Verification items for the finished model (mm, model axes). Face numbers are marked on the shaded views. A direction names the side the tool comes from. Round coordinates to 2 decimals unless told otherwise and drop trailing zeros. Loops run counter-clockwise (first coordinate to the right, second up) from the corner with the lowest first, then second, coordinate; pieces in that order, holes last. Notation, with made-up numbers: M -34.75,-4 L -15.75,-4 A25 cw -15.75,12 Z; hole C 34,-1.75 d11. An arc over 180 degrees is marked long. One line per item, written item: value.
from build123d import *

# Parameters (mm, degrees)
SKIZZE1_W                       = 60
SKIZZE1_H                       = 70
GRUNDK_RPER_DEPTH               = 20
FASE1_SIZE                      = 2
WANDUNG1_T                      = 3
SKIZZE2_R                       = 4.5
DURCHBRUCH_SERVO_DEPTH          = 100.13122616
SKIZZE4_W                       = 22
SKIZZE4_H                       = 42
SERVOFREISCHNITT_DEPTH          = 2
SKIZZE3_R                       = 2.1
FLANSCHAUFSATZ_DEPTH            = 6.5
SKIZZE6_R                       = 17.125
BOHRUNGSCHNECKE_DEPTH           = 6.5
SCHNITT_LINEAR_AUSTRAGEN2_REACH = 101.131
SKIZZE7_R                       = 2
SKIZZE8_R                       = 3.6
SCHNITT_LINEAR_AUSTRAGEN3_DEPTH = 2
FASE2_SIZE                      = 1
FASE3_SIZE                      = 0.5


with BuildPart() as part:
    # Skizze1 → Grundkörper (new body)
    with BuildSketch(Plane.XY):
        with Locations((30, 35)):
            Rectangle(SKIZZE1_W, SKIZZE1_H)
    extrude(amount=GRUNDK_RPER_DEPTH)

    # Fase1
    fase1_edges = [part.edges().sort_by_distance(p)[0] for p in [
        (0, 70, 10),
        (60, 70, 10),
        (60, 0, 10),
        (0, 0, 10),
    ]]
    chamfer(fase1_edges, length=FASE1_SIZE)

    # Wandung1
    wandung1_openings = [part.faces().sort_by_distance(p)[0] for p in [
        (30, 35, 0),
    ]]
    offset(amount=WANDUNG1_T, openings=wandung1_openings, kind=Kind.INTERSECTION)

    # Skizze2 → Durchbruch Servo (cut, through all)
    with BuildSketch(Plane.XY.offset(23)):
        with Locations((30, 24)):
            Circle(SKIZZE2_R)
    extrude(amount=-DURCHBRUCH_SERVO_DEPTH, mode=Mode.SUBTRACT)

    # Skizze4 → ServoFreischnitt (cut)
    with BuildSketch(Plane(origin=(0, 0, 20), x_dir=(-1, 0, 0), z_dir=(0, 0, -1))):
        with Locations((-30, 35)):
            Rectangle(SKIZZE4_W, SKIZZE4_H)
    extrude(amount=-SERVOFREISCHNITT_DEPTH, mode=Mode.SUBTRACT)

    # Skizze3 → FlanschAufsatz (add)
    with BuildSketch(Plane.XY.offset(23)):
        with BuildLine():
            Line((5, 31), (18.11121742, 38.820824834))
            ThreePointArc((18.11121742, 38.820824834), (30, 43), (41.88878258, 38.820824834))
            Line((41.88878258, 38.820824834), (55, 31))
            ThreePointArc((55, 31), (62, 24), (55, 17))
            Line((55, 17), (41.88878258, 9.179175166))
            ThreePointArc((41.88878258, 9.179175166), (30, 5), (18.11121742, 9.179175166))
            Line((18.11121742, 9.179175166), (5, 17))
            ThreePointArc((5, 17), (-2, 24), (5, 31))
        make_face()
        with Locations(Location((5, 24, 0), (0, 0, 180))):
            Circle(SKIZZE3_R, mode=Mode.SUBTRACT)
        with Locations(Location((55, 24, 0), (0, 0, 180))):
            Circle(SKIZZE3_R, mode=Mode.SUBTRACT)
    extrude(amount=FLANSCHAUFSATZ_DEPTH)

    # Skizze6 → BohrungSchnecke (cut)
    with BuildSketch(Plane.XY.offset(29.5)):
        with Locations((30, 24)):
            Circle(SKIZZE6_R)
    extrude(amount=-BOHRUNGSCHNECKE_DEPTH, mode=Mode.SUBTRACT)

    # Skizze7 → Schnitt-Linear austragen2 (cut, up to next)
    with BuildSketch(Plane.XY.offset(23), mode=Mode.PRIVATE) as schnitt_linear_austragen2_sk1:
        with Locations((8, 62)):
            Circle(SKIZZE7_R)
    schnitt_linear_austragen2_tool1 = extrude(schnitt_linear_austragen2_sk1.sketch, amount=-SCHNITT_LINEAR_AUSTRAGEN2_REACH, mode=Mode.PRIVATE) & part.part
    # Skizze7 → Schnitt-Linear austragen2 (cut, up to next)
    with BuildSketch(Plane.XY.offset(23), mode=Mode.PRIVATE) as schnitt_linear_austragen2_sk2:
        with Locations(Location((52, 62, 0), (0, 0, 180))):
            Circle(SKIZZE7_R)
    schnitt_linear_austragen2_tool2 = extrude(schnitt_linear_austragen2_sk2.sketch, amount=-SCHNITT_LINEAR_AUSTRAGEN2_REACH, mode=Mode.PRIVATE) & part.part
    # Skizze7 → Schnitt-Linear austragen2 (cut, up to next)
    with BuildSketch(Plane.XY.offset(23), mode=Mode.PRIVATE) as schnitt_linear_austragen2_sk3:
        with Locations((52, 8)):
            Circle(SKIZZE7_R)
    schnitt_linear_austragen2_tool3 = extrude(schnitt_linear_austragen2_sk3.sketch, amount=-SCHNITT_LINEAR_AUSTRAGEN2_REACH, mode=Mode.PRIVATE) & part.part
    # Skizze7 → Schnitt-Linear austragen2 (cut, up to next)
    with BuildSketch(Plane.XY.offset(23), mode=Mode.PRIVATE) as schnitt_linear_austragen2_sk4:
        with Locations(Location((8, 8, 0), (0, 0, 180))):
            Circle(SKIZZE7_R)
    schnitt_linear_austragen2_tool4 = extrude(schnitt_linear_austragen2_sk4.sketch, amount=-SCHNITT_LINEAR_AUSTRAGEN2_REACH, mode=Mode.PRIVATE) & part.part
    add(schnitt_linear_austragen2_tool1.solids().sort_by_distance((8, 62, 23))[0], mode=Mode.SUBTRACT)
    add(schnitt_linear_austragen2_tool2.solids().sort_by_distance((52, 62, 23))[0], mode=Mode.SUBTRACT)
    add(schnitt_linear_austragen2_tool3.solids().sort_by_distance((52, 8, 23))[0], mode=Mode.SUBTRACT)
    add(schnitt_linear_austragen2_tool4.solids().sort_by_distance((8, 8, 23))[0], mode=Mode.SUBTRACT)

    # Skizze8 → Schnitt-Linear austragen3 (cut)
    with BuildSketch(Plane.XY.offset(23)):
        with Locations((8, 62)):
            Circle(SKIZZE8_R)
        with Locations((52, 62)):
            Circle(SKIZZE8_R)
        with Locations((52, 8)):
            Circle(SKIZZE8_R)
        with Locations((8, 8)):
            Circle(SKIZZE8_R)
    extrude(amount=-SCHNITT_LINEAR_AUSTRAGEN3_DEPTH, mode=Mode.SUBTRACT)

    # Fase2
    fase2_edges = [part.edges().sort_by_distance(p)[0] for p in [
        (63, 35, 23),
        (30, -3, 23),
        (-3, 35, 23),
        (30, 73, 23),
        (61.121320344, 71.121320344, 23),
        (-1.121320344, 71.121320344, 23),
        (-1.121320344, -1.121320344, 23),
        (61.121320344, -1.121320344, 23),
    ]]
    chamfer(fase2_edges, length=FASE2_SIZE - 0.0001)  # a hair under: the kernel refuses the full size

    # Fase3
    fase3_edges = [part.edges().sort_by_distance(p)[0] for p in [
        (63, 35, 0),
        (-3, 35, 0),
        (30, 73, 0),
        (30, -3, 0),
        (61.121320344, 71.121320344, 0),
        (-1.121320344, 71.121320344, 0),
        (-1.121320344, -1.121320344, 0),
        (61.121320344, -1.121320344, 0),
        (0, 35, 0),
        (30, 0, 0),
        (60, 35, 0),
        (30, 70, 0),
        (59, 1, 0),
        (1, 1, 0),
        (1, 69, 0),
        (59, 69, 0),
    ]]
    chamfer(fase3_edges, length=FASE3_SIZE)


solid = part.part
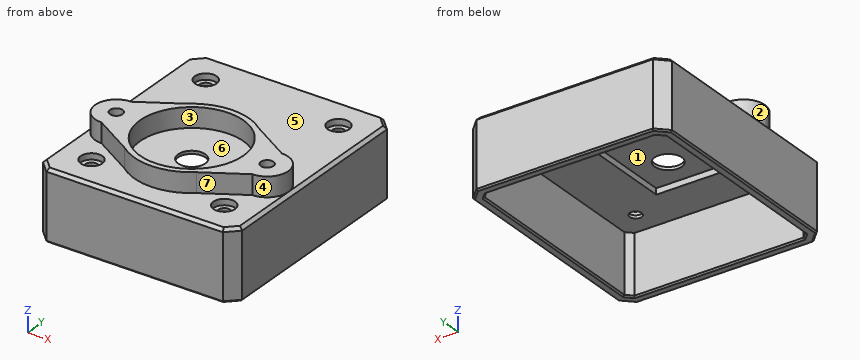
(1) Thickness scan on L1, parallel to Y at x = 8, z = 22; L2, parallel to Y at x = 55, z = 27; L3, parallel to X at y = 26, z = 12.5. Record the ranges inside material, lowest first. Write a range as from..to.
Completed:
L1: y = -3..4.4, 11.6..58.4, 65.6..73
L2: y = 17..21.9, 26.1..31
L3: x = -3..0, 60..63
(2) Sectioned sample at C-C on z = 27.75. Enter the section's corners in (x, y) (3 decimals).
Completed:
outline: M 5,17 L 18.111,9.179 A19 ccw 41.889,9.179 L 55,17 A7 ccw 55,31 L 41.889,38.821 A19 ccw 18.111,38.821 L 5,31 A7 ccw Z; hole C 5,24 d4.2; hole C 30,24 d34.25; hole C 55,24 d4.2
(3) Tool access check on the marked faces 1, 2, 3 and 4. Record the directions out of +Z, -Z, +X, -X, +Y, -Y that give a thin tool (end or side, any length) a straight path to the whole face; none if there is none.
Completed:
face 1: -Z
face 2: +Z, -X
face 3: +Z
face 4: +Z, +X
(4) Sectioned sample at B-B on y = 62. Count the separate pieces of the cut face and the enclosed holes in it, and give its area (3 significant figures).
Completed:
separate pieces: 3
enclosed holes: 0
area: 280 mm^2
(5) Depth check by flat-ended pin: pin 1 Ø6 at (x, y) = (9.5, 61.5) entering from +Z; pin 2 Ø3 at (x, y) = (8, 13) entering from -Z; pin 3 Ø11.5 at (x, y) = (30, 24) entering from -Z. Enter the tip coordinate at first touch or a pass-through.
Completed:
pin 1: stops at z = 23
pin 2: stops at z = 20
pin 3: stops at z = 22
(6) Mould release check, pull along Y, two halves, no side actions. Record for the marked faces 5, 6 and 7: +Y half, -Y half, draft (parallel to the pull), parting line (faces both ways), or undercut.
Completed:
face 5: draft
face 6: undercut
face 7: -Y half
